from build123d import *

# Parameters (mm, degrees)
SKETCH1_W               = 8
SKETCH1_H               = 8
BOSS_EXTRUDE1_DEPTH     = 3
CUT_EXTRUDE1_DEPTH      = 12.704699911
CUT_EXTRUDE1_DEPTH_BACK = 12.704699911
CUT_EXTRUDE2_DEPTH      = 11
SKETCH4_R               = 1.8
CUT_EXTRUDE3_DEPTH      = 0.8
SKETCH5_W               = 8
SKETCH5_H               = 1
BOSS_EXTRUDE2_DEPTH     = 2
FILLET1_R               = 4
CUT_EXTRUDE4_DEPTH      = 0.4
SKETCH7_W               = 1.384615385
SKETCH7_H               = 0.333333334
CUT_EXTRUDE5_DEPTH      = 0.4


with BuildPart() as part:
    # Sketch1 → Boss-Extrude1 (new body)
    with BuildSketch(Plane(origin=(0, 0, 0), x_dir=(1, 0, 0), z_dir=(0, 1, 0))):
        with Locations((4, 4)):
            Rectangle(SKETCH1_W, SKETCH1_H)
    extrude(amount=BOSS_EXTRUDE1_DEPTH)

    # Sketch2 → Cut-Extrude1 (cut, two sides: drawn at the far end of the back side and taken through both)
    with BuildSketch(Plane.XY.offset(-CUT_EXTRUDE1_DEPTH_BACK)):
        Polygon((0, 0), (0.6, 3), (0, 3), align=None)
        Polygon((8, 0), (7.4, 3), (8, 3), align=None)
    extrude(amount=CUT_EXTRUDE1_DEPTH + CUT_EXTRUDE1_DEPTH_BACK, mode=Mode.SUBTRACT)

    # Sketch3 → Cut-Extrude2 (cut)
    with BuildSketch(Plane(origin=(0, 0, 0), x_dir=(0, 0, -1), z_dir=(1, 0, 0))):
        Polygon((0, 0), (0.6, 3), (0, 3), align=None)
        Polygon((8, 3), (7.4, 3), (8, 0), align=None)
    extrude(amount=CUT_EXTRUDE2_DEPTH, mode=Mode.SUBTRACT)

    # Sketch4 → Cut-Extrude3 (cut)
    with BuildSketch(Plane.XZ):
        with Locations(Location((4, -3.75, 0), (0, 0, 270))):
            Circle(SKETCH4_R)
    extrude(amount=-CUT_EXTRUDE3_DEPTH, mode=Mode.SUBTRACT)

    # Sketch5 → Boss-Extrude2 (add)
    with BuildSketch(Plane.XZ):
        with Locations((4, -7.5)):
            Rectangle(SKETCH5_W, SKETCH5_H)
    extrude(amount=BOSS_EXTRUDE2_DEPTH)

    # Fillet1
    # the kernel refuses this fillet: 4 mm, written as the material it takes off along each edge
    with BuildSketch(Plane(origin=(8, -2, -16.660254038), x_dir=(0, 1, 0), z_dir=(0, 0, 1)), Plane(origin=(0, -2, 1.660254038), x_dir=(0, 1, 0), z_dir=(0, 0, -1))) as fillet1_piece_1:
        with BuildLine():
            CenterArc((4, 3.464101615), FILLET1_R, 180, 60)
            Line((0, 3.464101615), (-0.08, 3.464101615))
            Line((-0.08, 3.464101615), (-0.08, 0))
            Line((-0.08, 0), (0, -0.08))
            ThreePointArc((0, -0.08), (1, -0.08), (1.96, -0.069282032))
            Line((1.96, -0.069282032), (2, 0))
        make_face()
    extrude(amount=18.320508076, mode=Mode.SUBTRACT)

    # Sketch6 → Cut-Extrude4 (cut)
    with BuildSketch(Plane(origin=(0, 3, 0), x_dir=(1, 0, 0), z_dir=(0, 1, 0))):
        with BuildLine():
            Line((2.436272881, 5.979723732), (3.903420317, 5.979723732))
            add(Edge.make_bspline(
                [(3.903420317, 5.979723732), (3.943490496, 5.979744505), (4.021516441, 5.979784954), (4.134752515, 5.975087302), (4.240642802, 5.970362082), (4.338883372, 5.960903224), (4.429815049, 5.950988663), (4.51360101, 5.938436084), (4.589711972, 5.922348579), (4.637707501, 5.909661658), (4.660631856, 5.903601937)],
                knots=[0, 0, 0, 0, 1.259756885, 2.453039283, 3.563158368, 4.591894114, 5.55549294, 6.43918076, 7.254497783, 8, 8, 8, 8], degree=3))
            add(Edge.make_bspline(
                [(4.660631856, 5.903601937), (4.689300162, 5.894258489), (4.74612039, 5.87573989), (4.829420592, 5.843292221), (4.908343197, 5.803050568), (4.985816138, 5.760749105), (5.058380803, 5.710732544), (5.129877456, 5.658697008), (5.195666079, 5.598419283), (5.281939397, 5.514177193), (5.380383811, 5.396825298), (5.483519335, 5.241163905), (5.570813292, 5.070304112), (5.630456537, 4.917219685), (5.670729972, 4.787084992), (5.697056277, 4.682749965), (5.719418871, 4.572846322), (5.737778631, 4.457346355), (5.752043635, 4.336250048), (5.762664083, 4.209589679), (5.767837312, 4.07725583), (5.769008616, 3.987205692), (5.769606215, 3.941262194)],
                knots=[0, 0, 0, 0, 0.745524535, 1.477620414, 2.207090574, 2.934465325, 3.657932502, 4.384347339, 5.118673636, 5.861150177, 7.365375624, 8.894729774, 10.468936425, 12.099947606, 12.950091786, 13.83580991, 14.759228729, 15.722225242, 16.726454549, 17.773376212, 18.863978586, 20, 20, 20, 20], degree=3))
            add(Edge.make_bspline(
                [(5.769606215, 3.941262194), (5.768515323, 3.861857727), (5.766405561, 3.708291084), (5.741963835, 3.486695058), (5.70674022, 3.280872561), (5.667035899, 3.152471539), (5.647811343, 3.090300655)],
                knots=[0, 0, 0, 0, 1.103207939, 2.133582005, 3.096293362, 4, 4, 4, 4], degree=3))
            add(Edge.make_bspline(
                [(5.647811343, 3.090300655), (5.635116766, 3.054625647), (5.610144552, 2.98444734), (5.566445051, 2.883214788), (5.519227431, 2.786877042), (5.468100041, 2.695510004), (5.412804571, 2.609524646), (5.353134197, 2.529178156), (5.290013855, 2.453412746), (5.244286819, 2.406778778), (5.221529292, 2.383569886)],
                knots=[0, 0, 0, 0, 1.090884612, 2.145940218, 3.175104604, 4.181306866, 5.161203701, 6.118658341, 7.063689906, 8, 8, 8, 8], degree=3))
            add(Edge.make_bspline(
                [(5.221529292, 2.383569886), (5.184702113, 2.350450915), (5.108759222, 2.282154876), (4.974934842, 2.197635799), (4.823675662, 2.122952418), (4.714264019, 2.084588805), (4.657426727, 2.06465963)],
                knots=[0, 0, 0, 0, 0.908140292, 1.872714733, 2.8949153, 4, 4, 4, 4], degree=3))
            add(Edge.make_bspline(
                [(4.657426727, 2.06465963), (4.634546833, 2.057632533), (4.587060796, 2.043048157), (4.511767003, 2.027471741), (4.431388989, 2.011061834), (4.344999886, 2.001176252), (4.253496453, 1.990751469), (4.156149493, 1.984898536), (4.053296456, 1.980743294), (3.98275208, 1.980068625), (3.946689548, 1.979723732)],
                knots=[0, 0, 0, 0, 0.799129865, 1.658552685, 2.566799617, 3.538529252, 4.561352959, 5.643373779, 6.795284424, 8, 8, 8, 8], degree=3))
            Line((3.946689548, 1.979723732), (2.436272881, 1.979723732))
            Line((2.436272881, 1.979723732), (2.436272881, 5.979723732))
        make_face()
        with BuildLine():
            Line((3.205503651, 5.313057065), (3.205503651, 2.646390399))
            Line((3.205503651, 2.646390399), (3.838516471, 2.646390399))
            add(Edge.make_bspline(
                [(3.838516471, 2.646390399), (3.86709534, 2.646617049), (3.922120581, 2.647053436), (4.001743514, 2.648335709), (4.07491632, 2.651807064), (4.142022322, 2.655402822), (4.202886818, 2.661343643), (4.257774639, 2.667186667), (4.306380252, 2.675360935), (4.336400272, 2.681813595), (4.350535702, 2.684851937)],
                knots=[0, 0, 0, 0, 1.333384787, 2.567275092, 3.714769766, 4.750907381, 5.701951617, 6.567520054, 7.325492842, 8, 8, 8, 8], degree=3))
            add(Edge.make_bspline(
                [(4.350535702, 2.684851937), (4.38364248, 2.693686468), (4.44812575, 2.710893803), (4.538666782, 2.749253907), (4.62059475, 2.795531175), (4.695281698, 2.8511776), (4.762590099, 2.92150181), (4.820046047, 3.011440962), (4.873220012, 3.118706088), (4.909633556, 3.221385639), (4.935771128, 3.313096613), (4.95346412, 3.390071897), (4.967446413, 3.47335137), (4.979473009, 3.562606359), (4.989190784, 3.657722085), (4.995237644, 3.759042029), (4.999364663, 3.866442163), (5.000032135, 3.940189623), (5.000375445, 3.978121168)],
                knots=[0, 0, 0, 0, 1.038686998, 2.023088296, 2.974059649, 3.888265163, 4.839857954, 5.909819677, 7.113156087, 8.466843969, 9.20827164, 10.006482943, 10.861893492, 11.769681931, 12.739021491, 13.762258324, 14.849031541, 16, 16, 16, 16], degree=3))
            add(Edge.make_bspline(
                [(5.000375445, 3.978121168), (5.000034775, 4.01605283), (4.999374834, 4.089533605), (4.995254144, 4.196132914), (4.989241251, 4.29585735), (4.979454269, 4.38883019), (4.967614104, 4.475179926), (4.953468032, 4.554979633), (4.935881696, 4.627705609), (4.909721893, 4.71410541), (4.870064977, 4.811221472), (4.816099655, 4.917402921), (4.749828382, 5.00790436), (4.676605078, 5.08652444), (4.592177372, 5.151224792), (4.498716105, 5.205415106), (4.394186359, 5.247475499), (4.319831067, 5.2653904), (4.281625445, 5.274595527)],
                knots=[0, 0, 0, 0, 1.117996097, 2.165769068, 3.143980016, 4.062055362, 4.920439205, 5.712587309, 6.449616741, 7.124491204, 8.371470382, 9.537068822, 10.625202851, 11.666538334, 12.693249444, 13.747832046, 14.842779399, 16, 16, 16, 16], degree=3))
            add(Edge.make_bspline(
                [(4.281625445, 5.274595527), (4.265088191, 5.27766838), (4.228679487, 5.284433627), (4.168262747, 5.292335475), (4.097380449, 5.298199321), (4.015671249, 5.304185793), (3.923465993, 5.307602683), (3.820378875, 5.311168762), (3.706841263, 5.312386928), (3.627511913, 5.312827267), (3.586112625, 5.313057065)],
                knots=[0, 0, 0, 0, 0.578738571, 1.274160813, 2.095454135, 3.025967819, 4.093109015, 5.270126069, 6.575371698, 8, 8, 8, 8], degree=3))
            Line((3.586112625, 5.313057065), (3.205503651, 5.313057065))
        make_face(mode=Mode.SUBTRACT)
    extrude(amount=-CUT_EXTRUDE4_DEPTH, mode=Mode.SUBTRACT)

    # Sketch7 → Cut-Extrude5 (cut)
    with BuildSketch(Plane(origin=(0, 3, 0), x_dir=(1, 0, 0), z_dir=(0, 1, 0))):
        with Locations((6.167407218, 1.778686134)):
            Rectangle(SKETCH7_W, SKETCH7_H)
        with Locations((6.167407218, 1.188942544)):
            Rectangle(SKETCH7_W, SKETCH7_H)
    extrude(amount=-CUT_EXTRUDE5_DEPTH, mode=Mode.SUBTRACT)


solid = part.part
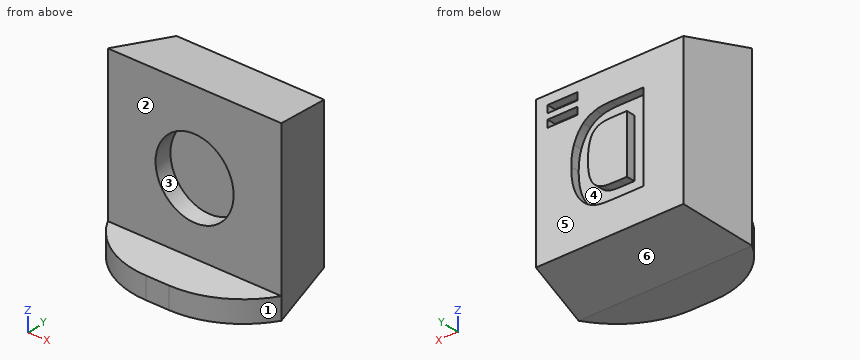
Could you check a few things on this model? Use its own coordinates, in mm. Face numbers are marked on the shaded views. A direction names the side the tool comes from. Give positions to 0.01 mm unless a question says otherwise; leave off trailing zeros. Loops run counter-clockwise (first coordinate to the right, second up) from the corner with the lowest first, then second, coordinate; pieces in that order, holes last. Notation, with made-up numbers: (-33, 74.25) -> (22, 74.25) arc R22 cw to (22, 111.25) -> close; hole circle Ø7 at (-17.5, -38.5). An arc over 180 degrees is marked (long way). Answer as CSV lines item,"result". Start each with the question number.
(1) If we section it at A-A on y = 0.35: Write out the boundary of the cut face in (x, z), then the cut area to 3 significant figures.
(2) I need wall thicknesses on probe 1 along Y at (x, z) = (6, -6.5); probe 2 along Y at (x, z) = (3, -5.75); probe 3 along X at (y, z) = (0.45, -3.75). Which ranges of each line are inside material? Lowest first, please.
(3) I'm going to push flat-ended pins straight in: pin 1 Ø1.5 at (y, z) = (-1, -5.5) entering from -X; pin 2 Ø3 at (x, z) = (4, -3) entering from -Y; pin 3 Ø1 at (y, z) = (2, -1.5) entering from -X. Where does each tip first touch, or does it pass through?
(4) We'd pull the mould along Z, two halves only. Please class the marked faces 4, 5 and 6: released by +Z, released by -Z, zero draft, split by the parting line, or undercut.
(5) If we section it at D-D on y = -1.15: Write out the boundary of the cut face in (x, z), then the cut area to 3 significant figures.
(6) If we section it at C-C on x = 1.75: Write out the boundary of the cut face in (y, z).
(7) Which directions (+Z, -Z, +X, -X, +Y, -Y) give clear straight access to the entire face, cutting with the end or side of a thin tool? Please do the marked faces 1, 2 and 3.
(8) If we section it at B-B on y = 1.35: Write out the boundary of the cut face in (x, z), then the cut area to 3 significant figures.
Computed:
1,outline,"(0.07, -7.93) -> (7.93, -7.93) -> (7.93, -0.07) -> (0.07, -0.07) -> close; hole circle Ø3.6 at (4, -3.75)"
1,area,"51.6 mm2"
2,probe 1,"y = 0 to 3"
2,probe 2,"y = 0 to 2.6"
2,probe 3,"x = 0.09 to 2.2, 5.8 to 7.91"
3,pin 1,"passes through"
3,pin 2,"stops at y = 0"
3,pin 3,"stops at x = 0.3"
4,face 4,"undercut"
4,face 5,"zero draft"
4,face 6,"released by -Z"
5,outline,"(1, -8) -> (7, -8) -> (7, -7) -> (1, -7) -> close"
5,area,"6.00 mm2"
6,outline,"(-1.61, -8) -> (0, -8) -> (3, -7.4) -> (3, -0.6) -> (0, 0) -> (0, -7) -> (-1.61, -7) -> close"
7,face 1,"+Z, -Z, +X, -Y"
7,face 2,"+Z, +X, -X, -Y"
7,face 3,"-Y"
8,outline,"(0.27, -7.73) -> (7.73, -7.73) -> (7.73, -0.27) -> (0.27, -0.27) -> close"
8,area,"55.7 mm2"
